Design review of the part built by this model. Coordinates are the model's own, in mm. A direction names the side the tool comes from. Coordinates: 2 decimals unless noted, no trailing zeros. Order: outer loops, then holes, each group sorted by start corner. A loop starts at its lowest first (then second) coordinate and runs counter-clockwise, first axis right, second up. Notation, with made-up numbers: M -23,12.25 L 9,12.25 A23 cw 9,30.25 Z; hole C -26,55 d10. An arc over 180 degrees is marked long. Answer in a Markdown table with one row per item.
from build123d import *

# Parameters (mm, degrees)
SKETCH_W        = 90
SKETCH_H        = 40
PAD_DEPTH       = 10
SKETCH001_R     = 6
SKETCH001_R_2   = 2.5
POCKET_DEPTH    = 10.001
SKETCH002_R     = 4
POCKET001_DEPTH = 5
SKETCH004_R     = 11
POCKET003_DEPTH = 7


with BuildPart() as part:
    # Sketch → Pad (new body)
    with BuildSketch(Plane.XY):
        Rectangle(SKETCH_W, SKETCH_H)
    extrude(amount=PAD_DEPTH)

    # Sketch001 (on Face6 of Pad) → Pocket (cut, through all)
    with BuildSketch(Plane.XY.offset(10)):
        with Locations((0, 7)):
            Circle(SKETCH001_R)
        with Locations((-30, -10)):
            Circle(SKETCH001_R_2)
        with Locations((30, -10)):
            Circle(SKETCH001_R_2)
    extrude(amount=-POCKET_DEPTH, mode=Mode.SUBTRACT)

    # Sketch002 (on Face5 of Pocket) → Pocket001 (cut)
    with BuildSketch(Plane.XY.offset(10)):
        with Locations((30, -10)):
            Circle(SKETCH002_R)
        with Locations((0, 7)):
            Circle(SKETCH002_R)
        with Locations((-30, -10)):
            Circle(SKETCH002_R)
    extrude(amount=-POCKET001_DEPTH, mode=Mode.SUBTRACT)

    # Sketch004 (on Face4 of Pocket001) → Pocket003 (cut)
    with BuildSketch(Plane(origin=(0, 0, 0), x_dir=(1, 0, 0), z_dir=(0, 0, -1))):
        with Locations((0, -7)):
            Circle(SKETCH004_R)
    extrude(amount=-POCKET003_DEPTH, mode=Mode.SUBTRACT)


solid = part.part
(1) For line 1 along Y through (x, z) = (30, 3.5); line 2 along Y through (x, z) = (0, 9.25); line 3 along X through (y, z) = (-7, 7.25), list the stretches that pass through material, from the lowest coordinate up. Write a range as from..to.
Return value:
| item | result |
|---|---|
| line 1 | y = -20..-12.5, -7.5..20 |
| line 2 | y = -20..1, 13..20 |
| line 3 | x = -45..-32.65, -27.35..27.35, 32.65..45 |
(2) Draft analysis for pull direction X (two halves, no side actions). For faces 4 (the flat face through (5, 12, 7)), 5 (the cylindrical face through (26.8, -12.4, 7.5)), 6 (the flat face through (-0.6, -4.2, 0)), 7 (the flat face through (-45, 0, 5)), state which applies: pulls with the +X half, pulls with the -X half, needs draft (parallel to the pull), parting line crosses it, or undercut.
Return value:
| item | result |
|---|---|
| face 4 | undercut |
| face 5 | undercut |
| face 6 | needs draft |
| face 7 | pulls with the -X half |
(3) Add section B-B, the plane z = 1.25. Give the boundary of the cut face in (x, y), and give its area (3 significant figures).
Return value:
| item | result |
|---|---|
| outline | M -45,-20 L 45,-20 L 45,20 L -45,20 Z; hole C -30,-10 d5; hole C 0,7 d22; hole C 30,-10 d5 |
| area | 3,180 mm2 |
(4) Insertion check: pin 1 Ø10 at (x, y) = (-18.5, 2) entering from -Z; pin 2 Ø6.5 at (x, y) = (-3.5, 6.5) entering from -Z; pin 3 Ø6.5 at (x, y) = (30, -10) entering from +Z. Each pin has a flat end and moves straight along its axis. Give the tip position at first contact, or say it passes through.
Return value:
| item | result |
|---|---|
| pin 1 | stops at z = 0 |
| pin 2 | stops at z = 7 |
| pin 3 | stops at z = 5 |
(5) For faces 1 (the cylindrical face through (-2.38, 17.74, 3.45)), 2 (the flat face through (-1, 20, 5)), 3 (the flat face through (-28, -8, 5)), list the 3-axis set-ups (+Z, -Z, +X, -X, +Y, -Y) from which the entire face can be reached by the end or side of a thin tool; tool diameter is ignored.
Return value:
| item | result |
|---|---|
| face 1 | -Z |
| face 2 | +Z, -Z, +X, -X, +Y |
| face 3 | +Z |
(6) Add section A-A, the plane y = -10. Give the boundary of the cut face in (x, z).
Return value:
| item | result |
|---|---|
| outline | M -45,0 L -32.5,0 L -32.5,5 L -34,5 L -34,10 L -45,10 Z; M -27.5,0 L 27.5,0 L 27.5,5 L 26,5 L 26,10 L -26,10 L -26,5 L -27.5,5 Z; M 32.5,0 L 45,0 L 45,10 L 34,10 L 34,5 L 32.5,5 Z |
(7) Add section C-C, the plane x = 30. Give the boundary of the cut face in (y, z), and give its area (3 significant figures).
Return value:
| item | result |
|---|---|
| outline | M -20,0 L -12.5,0 L -12.5,5 L -14,5 L -14,10 L -20,10 Z; M -7.5,0 L 20,0 L 20,10 L -6,10 L -6,5 L -7.5,5 Z |
| area | 335 mm2 |
(8) Add section D-D, the plane y = 7. Give the boundary of the cut face in (x, z), and give its area (3 significant figures).
Return value:
| item | result |
|---|---|
| outline | M -45,0 L -11,0 L -11,7 L -6,7 L -6,10 L -45,10 Z; M 6,7 L 11,7 L 11,0 L 45,0 L 45,10 L 6,10 Z |
| area | 710 mm2 |
